Read the model definition and answer for the solid it produces. Units are mm, in the model's axes. A direction names the side the tool comes from. Coordinates: 2 decimals unless noted, no trailing zeros. Order: outer loops, then holes, each group sorted by start corner. A loop starts at its lowest first (then second) coordinate and runs counter-clockwise, first axis right, second up.
Autodesk Inventor part; units mm, degrees
ref_plane "YZ Plane" through (0, 0, 0) normal (1, 0, 0) x (0, 1, 0)
ref_plane "XZ Plane" through (0, 0, 0) normal (0, 1, 0) x (-1, 0, 0)
ref_plane "XY Plane" through (0, 0, 0) normal (0, 0, 1) x (1, 0, 0)
sketch "Sketch1" plane through (0, 0, 0) normal (0, 0, 1) x (1, 0, 0)
  circle A0 centre (0, 0) radius 16
  dimension "d0" = 32
extrude "Extrusion1" add sketch "Sketch1" along normal blind 6
sketch "Sketch2" plane through (0, 0, 6) normal (0, 0, 1) x (1, 0, 0)
  circle A0 centre (-10.3923, -6) radius 2.5
  circle A1 centre (10.3923, -6) radius 2.5
  circle A2 centre (0, 0) radius 12 construction
  line L0 (-10.3923, -6) -> (0, 0) construction
  line L1 (0, 0) -> (10.3923, -6) construction
  line L2 (0, 0) -> (0, 12) construction
  dimension "d3" = 120
  dimension "d4" = 5
  dimension "d5" = 24
sketch "Sketch3" plane through (0, 0, 6) normal (0, 0, 1) x (1, 0, 0)
  circle A0 centre (0, 0) radius 1.5
  circle A1 centre (0, 6.35) radius 1.5
  circle A2 centre (0, 0) radius 6.35 construction
  circle A3 centre (-6.35, 0) radius 1.5
  circle A4 centre (0, -6.35) radius 1.5
  circle A5 centre (6.35, 0) radius 1.5
  dimension "d8" = 3
  dimension "d13" = 3
  dimension "d14" = 6.35
  dimension "d17" = 360
extrude "Extrusion3" cut sketch "Sketch3" against normal up to next
extrude "Extrusion4" cut sketch "Sketch2" against normal blind 2
properties part number "slider_wheel"
1) Which of the six approach directions +Z, -Z, +X, -X, +Y, -Y give full straight-line access (tool end or side, diameter ignored) to faces 1 (the cylindrical face through (-4.964, -0.575, 3.042)), 2 (the cylindrical face through (7.895, -5.89, 5.014))?
A:
face 1: +Z, -Z
face 2: +Z
2) A cutting plane is placed at D-D, the plane z = 2.8. Determine the outline of the cut face in (x, y).
A:
outline: circle Ø32 at (0, 0); hole circle Ø3 at (-6.35, 0); hole circle Ø3 at (0, -6.35); hole circle Ø3 at (0, 0); hole circle Ø3 at (0, 6.35); hole circle Ø3 at (6.35, 0)
3) A cutting plane is placed at A-A, the plane y = 0. Determine the outline of the cut face in (x, z), and give its area (3 significant figures).
A:
outline: (-16, 0) - (-7.85, 0) - (-7.85, 6) - (-16, 6) - close; (-4.85, 0) - (-1.5, 0) - (-1.5, 6) - (-4.85, 6) - close; (1.5, 0) - (4.85, 0) - (4.85, 6) - (1.5, 6) - close; (7.85, 0) - (16, 0) - (16, 6) - (7.85, 6) - close
area: 138 mm2
4) A cutting plane is placed at B-B, the plane x = 6.35. Determine the outline of the cut face in (y, z), and give its area (3 significant figures).
A:
outline: (-14.69, 0) - (-1.5, 0) - (-1.5, 6) - (-14.69, 6) - close; (1.5, 0) - (14.69, 0) - (14.69, 6) - (1.5, 6) - close
area: 158 mm2
5) Flat-ended cylindrical pins translate along their axes: pin 1 Ø1.8 at (x, y) = (0, -6.35) entering from +Z; pin 2 Ø2.5 at (x, y) = (-10.5, -5) entering from +Z; pin 3 Ø1 at (y, z) = (-1.5, 5) entering from +X. Find the tip coordinate at first contact, or state that the pin passes through.
A:
pin 1: passes through
pin 2: stops at z = 4
pin 3: stops at x = 15.97
6) Determine the mould class of faces 3 (the cylindrical face through (-12.235, -4.31, 5.014)), 4 (the cylindrical face through (-3.47, 15.62, 2.96)), 5 (the flat face through (3, 0, 6)), 6 (the cylindrical face through (-0.195, -4.863, 3.042)) for opening direction Y: pulls with the +Y half, pulls with the -Y half, needs draft (parallel to the pull), parting line crosses it, or undercut.
A:
face 3: undercut
face 4: parting line crosses it
face 5: needs draft
face 6: undercut
7) Straight lines are drawn through the part: line 1 (Y direction, x = 0, z = 4.5); line 2 (Z direction, x = 8.5, y = -7); line 3 (X direction, y = 1, z = 3.25). For each, find the intervals that lie inside material, in ascending order.
A:
line 1: y = -16 to -7.85, -4.85 to -1.5, 1.5 to 4.85, 7.85 to 16
line 2: z = 0 to 4
line 3: x = -15.97 to -7.47, -5.23 to -1.12, 1.12 to 5.23, 7.47 to 15.97
